```python
from build123d import *

# Parameters (mm, degrees)
CROQUIS1_R              = 4.2
SALIENTE_EXTRUIR1_DEPTH = 4
SALIENTE_EXTRUIR2_DEPTH = 4
CROQUIS2_3_R            = 4.2
CORTAR_EXTRUIR1_DEPTH   = 4


with BuildPart() as part:
    # Croquis1 → Saliente-Extruir1 (new body)
    with BuildSketch(Plane.XY):
        with BuildLine():
            Line((2, 14.378089444), (-2, 14.378089444))
            Line((-2, 14.378089444), (-2, -5.621910556))
            Line((-2, -5.621910556), (2, -5.621910556))
            Line((2, -5.621910556), (2, -7.681185842))
            Line((2, -7.681185842), (20.292265124, -5.621910556))
            ThreePointArc((20.292265124, -5.621910556), (30.276145575, 4.378089444), (20.292265124, 14.378089444))
            Line((20.292265124, 14.378089444), (2, 16.43736473))
            Line((2, 16.43736473), (2, 14.378089444))
        make_face()
        with Locations((20.276132562, 4.378089444)):
            Circle(CROQUIS1_R, mode=Mode.SUBTRACT)
    extrude(amount=SALIENTE_EXTRUIR1_DEPTH)

    # Croquis2 → Saliente-Extruir2 (add)
    with BuildSketch(Plane.XY.offset(4)):
        with BuildLine():
            ThreePointArc((10.23085334, -6.754586935), (35.270935596, 4.378089444), (10.23085334, 15.510765823))
            Line((10.23085334, 15.510765823), (16.704250968, 14.782014755))
            ThreePointArc((16.704250968, 14.782014755), (26.667896891, 13.33048291), (31.276132562, 4.378089444))
            ThreePointArc((31.276132562, 4.378089444), (26.667896891, -4.574304022), (16.704250968, -6.025835867))
            Line((16.704250968, -6.025835867), (10.23085334, -6.754586935))
        make_face()
    extrude(amount=-SALIENTE_EXTRUIR2_DEPTH)

    # Croquis2_3 → Cortar-Extruir1 (cut)
    with BuildSketch(Plane.XY.offset(4)):
        with BuildLine():
            ThreePointArc((16.704250968, 14.782014755), (15.618415295, 14.343312465), (14.585373454, 13.791657353))
            ThreePointArc((14.585373454, 13.791657353), (9.276534219, 4.472091013), (14.425321372, -4.936845253))
            ThreePointArc((14.425321372, -4.936845253), (15.533426587, -5.546966729), (16.704250968, -6.025835867))
            Line((16.704250968, -6.025835867), (20.292265124, -5.621910556))
            ThreePointArc((20.292265124, -5.621910556), (30.276145575, 4.378089444), (20.292265124, 14.378089444))
            Line((20.292265124, 14.378089444), (16.704250968, 14.782014755))
        make_face()
        with Locations((20.276132562, 4.378089444)):
            Circle(CROQUIS2_3_R, mode=Mode.SUBTRACT)
    extrude(amount=-CORTAR_EXTRUIR1_DEPTH, mode=Mode.SUBTRACT)


solid = part.part
```
Geometry check sheet. Reference: the model listing, model coordinates, mm. A direction names the side the tool comes from. Round coordinates to 2 decimals unless told otherwise and drop trailing zeros. Order: outer loops, then holes, each group sorted by start corner. A loop starts at its lowest first (then second) coordinate and runs counter-clockwise, first axis right, second up. Notation, with made-up numbers: (17, -2.75) - (36, -2.75) arc R33 ccw to (36, 33.25) - close; hole circle Ø7 at (-10.75, -4). An arc over 180 degrees is marked (long way). Use a Markdown table: item, result. Add a question column.
1) Section check B-B (z = 0.7). Record the cut outline in (x, y), then the cut area to 3 significant figures.
2) Gauge pin test, flat ends, axial feed: P1, Ø1, axis at y = 16.5, z = 0.5, coming from the -X side; P2, Ø3, axis at x = 11, y = 3, coming from the -Z side. Record the tip position at first contact, or that the pin passes through.
3) Section check A-A (y = -1). Record the cut outline in (x, z).
4) Set-up check for faces 4 (the flat face through (0, 14.378, 2)), 5 (the flat face through (8, 5, 0)), 6 (the flat face through (6.173, 15.968, 1.972)): record each of +Z, -Z, +X, -X, +Y, -Y from which the full face is reachable in a straight line by a thin tool's end or side.
5) Thickness scan on line 1 along Y through (x, z) = (26, 1.95); line 2 along X through (y, z) = (-3.25, 2.85); line 3 along X through (y, z) = (-3, 2.4). Record the ranges inside material, lowest first.
6) Section check C-C (x = 21). Record the cut outline in (y, z).
7) Mould release check, pull along X, two halves, no side actions. Record for faces 1 (the flat face through (2, -7, 2)), 2 (the flat face through (6.058, -7.224, 1.972)), 3 (the flat face through (0, -5.622, 2)): released by +X, released by -X, zero draft, split by the parting line, or undercut.
Established:
| question | item | result |
|---|---|---|
| 1 | outline | (-2, -5.62) - (2, -5.62) - (2, -7.68) - (10.23, -6.75) arc R14.99 ccw (long way) to (10.23, 15.51) - (2, 16.44) - (2, 14.38) - (-2, 14.38) - close; hole circle Ø22 at (20.28, 4.38) |
| 1 | area | 521 mm2 |
| 2 | P1 | x = 2 |
| 2 | P2 | through |
| 3 | outline | (-2, 0) - (10.68, 0) - (10.68, 4) - (-2, 4) - close; (29.87, 0) - (34.27, 0) - (34.27, 4) - (29.87, 4) - close |
| 4 | face 4 | +Z, -Z, -X, +Y |
| 4 | face 5 | -Z, +X, -X, +Y, -Y |
| 4 | face 6 | +Z, -Z, +Y |
| 5 | line 1 | -9.48 to -5.02, 13.77 to 18.24 |
| 5 | line 2 | -2 to 12.35, 28.2 to 33.19 |
| 5 | line 3 | -2 to 12.12, 28.43 to 33.33 |
| 6 | outline | (-10.6, 0) - (-6.6, 0) - (-6.6, 4) - (-10.6, 4) - close; (15.35, 0) - (19.36, 0) - (19.36, 4) - (15.35, 4) - close |
| 7 | face 1 | released by -X |
| 7 | face 2 | undercut |
| 7 | face 3 | zero draft |
